Can you work these out from the model? Positions are in its coordinate system, mm. A direction names the side the tool comes from. Coordinates: 2 decimals unless noted, no trailing zeros. Loops run counter-clockwise (first coordinate to the right, second up) from the corner with the lowest first, then second, coordinate; pieces in that order, holes last.
```python
from build123d import *

# Parameters (mm, degrees)
EXTRUDE_1_DEPTH     = 5
SKETCH_2_W          = 3
SKETCH_2_H          = 10
SKETCH_2_H_2        = 20
SKETCH_2_H_3        = 12.022353437
CUT_EXTRUDE_1_DEPTH = 112.915146428
EXTRUDE_2_DEPTH     = 5
SKETCH_4_R          = 1.6
CUT_EXTRUDE_2_DEPTH = 114.705760628
SKETCH_5_R          = 1
CUT_EXTRUDE_3_DEPTH = 114.705760628


with BuildPart() as part:
    # 草图1 → 凸台-拉伸1 (new body)
    with BuildSketch(Plane.XY):
        Polygon((0, 0), (0, 100), (-25, 100), (-50, 0), align=None)
    extrude(amount=EXTRUDE_1_DEPTH)

    # 草图2 → 切除-拉伸1 (cut, through all)
    with BuildSketch(Plane.XY.offset(5)):
        with Locations((-1.5, 5)):
            Rectangle(SKETCH_2_W, SKETCH_2_H)
        with Locations((-1.5, 35)):
            Rectangle(SKETCH_2_W, SKETCH_2_H_2)
        with Locations((-1.5, 70)):
            Rectangle(SKETCH_2_W, SKETCH_2_H_2)
        with Locations((-1.5, 101.011176718)):
            Rectangle(SKETCH_2_W, SKETCH_2_H_3)
    extrude(amount=-CUT_EXTRUDE_1_DEPTH, mode=Mode.SUBTRACT)

    # 草图3 → 凸台-拉伸2 (add)
    with BuildSketch(Plane.XY.offset(5)):
        Polygon((-3, 100), (-3, 102), (-24.5, 102), (-25, 100), align=None)
    extrude(amount=-EXTRUDE_2_DEPTH)

    # 草图4 → 切除-拉伸2 (cut, through all)
    with BuildSketch(Plane.XY.offset(5)):
        with Locations((-25.157670781, 87)):
            Circle(SKETCH_4_R)
        with Locations((-43.157670781, 15)):
            Circle(SKETCH_4_R)
    extrude(amount=-CUT_EXTRUDE_2_DEPTH, mode=Mode.SUBTRACT)

    # 草图5 → 切除-拉伸3 (cut, through all)
    with BuildSketch(Plane.XY.offset(5)):
        with Locations((-2, 87.5)):
            Circle(SKETCH_5_R)
        with Locations((-2, 52.5)):
            Circle(SKETCH_5_R)
        with Locations((-2, 17.5)):
            Circle(SKETCH_5_R)
    extrude(amount=-CUT_EXTRUDE_3_DEPTH, mode=Mode.SUBTRACT)


solid = part.part
```
(1) I want a section at D-D on y = 93. Write out the boundary of the cut face in (x, z), then the cut area to 3 significant figures.
Check values:
outline: (-26.75, 0) - (0, 0) - (0, 5) - (-26.75, 5) - close
area: 134 mm2
(2) I'm going to push flat-ended pins straight in: pin 1 (0.9 mm diameter, centred on x = -2, z = 2, fed in from +Y); pin 2 (1.5 mm diameter, centred on y = 99.5, z = 3, fed in from +X); pin 3 (1.2 mm diameter, centred on x = -2, y = 52.5, fed in from +Z); pin 4 (1 mm diameter, centred on y = 37.5, z = 1.5, fed in from -X). Where does each tip first touch, or does it pass through?
Check values:
pin 1: stops at y = 95
pin 2: stops at x = -3
pin 3: passes through
pin 4: stops at x = -40.75
(3) I want a section at B-B on y = 15. Write out the boundary of the cut face in (x, z).
Check values:
outline: (-46.25, 0) - (-44.76, 0) - (-44.76, 5) - (-46.25, 5) - close; (-41.56, 0) - (0, 0) - (0, 5) - (-41.56, 5) - close
(4) I want a section at C-C on z = 3.6. Write out the boundary of the cut face in (x, y), then the cut area to 3 significant figures.
Check values:
outline: (-50, 0) - (-3, 0) - (-3, 10) - (0, 10) - (0, 25) - (-3, 25) - (-3, 45) - (0, 45) - (0, 60) - (-3, 60) - (-3, 80) - (0, 80) - (0, 95) - (-3, 95) - (-3, 102) - (-24.5, 102) - close; hole circle Ø3.2 at (-43.16, 15); hole circle Ø3.2 at (-25.16, 87); hole circle Ø2 at (-2, 17.5); hole circle Ø2 at (-2, 52.5); hole circle Ø2 at (-2, 87.5)
area: 3,600 mm2
(5) I want a section at A-A on x = -2. Write out the boundary of the cut face in (y, z).
Check values:
outline: (10, 0) - (16.5, 0) - (16.5, 5) - (10, 5) - close; (18.5, 0) - (25, 0) - (25, 5) - (18.5, 5) - close; (45, 0) - (51.5, 0) - (51.5, 5) - (45, 5) - close; (53.5, 0) - (60, 0) - (60, 5) - (53.5, 5) - close; (80, 0) - (86.5, 0) - (86.5, 5) - (80, 5) - close; (88.5, 0) - (95, 0) - (95, 5) - (88.5, 5) - close
(6) If I drill on probe 1 along Y at (x, z) = (-2, 1.8); probe 2 along X at (y, z) = (87.5, 3.55) (3 decimals); probe 3 along X at (y, z) = (87, 1.75), over which ranges is the centre line in solid material (lowest first)?
Check values:
probe 1: y = 10 to 16.5, 18.5 to 25, 45 to 51.5, 53.5 to 60, 80 to 86.5, 88.5 to 95
probe 2: x = -28.125 to -26.678, -23.638 to -3, -1 to 0
probe 3: x = -28.25 to -26.76, -23.56 to -2.87, -1.13 to 0
(7) Which directions (+Z, -Z, +X, -X, +Y, -Y) give clear straight access to the entire face, cutting with the end or side of a thin tool? Please do faces 1 (the flat face through (-27, 0, 2)), 2 (the flat face through (-3, 35, 3)), 3 (the flat face through (-2, 10, 3)), 4 (the flat face through (-3, 98, 3)).
Check values:
face 1: +Z, -Z, +X, -X, -Y
face 2: +Z, -Z, +X
face 3: +Z, -Z, +X, -Y
face 4: +Z, -Z, +X, +Y
(8) If we mould it in two halves opening along X, with no side actions, what happens to faces 5 (the flat face through (0, 17, 2)), 6 (the flat face through (-2, 95, 3)), 7 (the cylindrical face through (-1.54, 86.61, 2.54))? For each: released by +X, released by -X, zero draft, split by the parting line, or undercut.
Check values:
face 5: released by +X
face 6: zero draft
face 7: undercut
